from build123d import *

# Parameters (mm, degrees)
SKETCH_1_W          = 290
SKETCH_1_H          = 150
EXTRUDE_1_DEPTH     = 5
CUT_EXTRUDE_2_REACH = 165.325
SKETCH_5_R          = 27.5
SKETCH_5_R_2        = 2.6
FILLET_1_R          = 10
SKETCH_6_R          = 2.75
CUT_EXTRUDE_3_DEPTH = 10
SKETCH_7_R          = 1.6
CUT_EXTRUDE_4_DEPTH = 10


with BuildPart() as part:
    # 草图1 → 凸台-拉伸1 (new body)
    with BuildSketch(Plane.XY):
        Rectangle(SKETCH_1_W, SKETCH_1_H)
    extrude(amount=EXTRUDE_1_DEPTH)

    # 草图5 → 切除-拉伸2 (cut, up to next)
    with BuildSketch(Plane(origin=(0, 0, 0), x_dir=(-1, 0, 0), z_dir=(0, 0, -1)), mode=Mode.PRIVATE) as cut_extrude_2_sk1:
        Circle(SKETCH_5_R)
    cut_extrude_2_tool1 = extrude(cut_extrude_2_sk1.sketch, amount=-CUT_EXTRUDE_2_REACH, mode=Mode.PRIVATE) & part.part
    # 草图5 → 切除-拉伸2 (cut, up to next)
    with BuildSketch(Plane(origin=(0, 0, 0), x_dir=(-1, 0, 0), z_dir=(0, 0, -1)), mode=Mode.PRIVATE) as cut_extrude_2_sk2:
        with Locations((23.864853865, 23.864853865)):
            Circle(SKETCH_5_R_2)
    cut_extrude_2_tool2 = extrude(cut_extrude_2_sk2.sketch, amount=-CUT_EXTRUDE_2_REACH, mode=Mode.PRIVATE) & part.part
    # 草图5 → 切除-拉伸2 (cut, up to next)
    with BuildSketch(Plane(origin=(0, 0, 0), x_dir=(-1, 0, 0), z_dir=(0, 0, -1)), mode=Mode.PRIVATE) as cut_extrude_2_sk3:
        with Locations((0, 33.75)):
            Circle(SKETCH_5_R_2)
    cut_extrude_2_tool3 = extrude(cut_extrude_2_sk3.sketch, amount=-CUT_EXTRUDE_2_REACH, mode=Mode.PRIVATE) & part.part
    # 草图5 → 切除-拉伸2 (cut, up to next)
    with BuildSketch(Plane(origin=(0, 0, 0), x_dir=(-1, 0, 0), z_dir=(0, 0, -1)), mode=Mode.PRIVATE) as cut_extrude_2_sk4:
        with Locations((-23.864853865, 23.864853865)):
            Circle(SKETCH_5_R_2)
    cut_extrude_2_tool4 = extrude(cut_extrude_2_sk4.sketch, amount=-CUT_EXTRUDE_2_REACH, mode=Mode.PRIVATE) & part.part
    # 草图5 → 切除-拉伸2 (cut, up to next)
    with BuildSketch(Plane(origin=(0, 0, 0), x_dir=(-1, 0, 0), z_dir=(0, 0, -1)), mode=Mode.PRIVATE) as cut_extrude_2_sk5:
        with Locations((-33.75, 0)):
            Circle(SKETCH_5_R_2)
    cut_extrude_2_tool5 = extrude(cut_extrude_2_sk5.sketch, amount=-CUT_EXTRUDE_2_REACH, mode=Mode.PRIVATE) & part.part
    # 草图5 → 切除-拉伸2 (cut, up to next)
    with BuildSketch(Plane(origin=(0, 0, 0), x_dir=(-1, 0, 0), z_dir=(0, 0, -1)), mode=Mode.PRIVATE) as cut_extrude_2_sk6:
        with Locations((-23.864853865, -23.864853865)):
            Circle(SKETCH_5_R_2)
    cut_extrude_2_tool6 = extrude(cut_extrude_2_sk6.sketch, amount=-CUT_EXTRUDE_2_REACH, mode=Mode.PRIVATE) & part.part
    # 草图5 → 切除-拉伸2 (cut, up to next)
    with BuildSketch(Plane(origin=(0, 0, 0), x_dir=(-1, 0, 0), z_dir=(0, 0, -1)), mode=Mode.PRIVATE) as cut_extrude_2_sk7:
        with Locations((0, -33.75)):
            Circle(SKETCH_5_R_2)
    cut_extrude_2_tool7 = extrude(cut_extrude_2_sk7.sketch, amount=-CUT_EXTRUDE_2_REACH, mode=Mode.PRIVATE) & part.part
    # 草图5 → 切除-拉伸2 (cut, up to next)
    with BuildSketch(Plane(origin=(0, 0, 0), x_dir=(-1, 0, 0), z_dir=(0, 0, -1)), mode=Mode.PRIVATE) as cut_extrude_2_sk8:
        with Locations((23.864853865, -23.864853865)):
            Circle(SKETCH_5_R_2)
    cut_extrude_2_tool8 = extrude(cut_extrude_2_sk8.sketch, amount=-CUT_EXTRUDE_2_REACH, mode=Mode.PRIVATE) & part.part
    # 草图5 → 切除-拉伸2 (cut, up to next)
    with BuildSketch(Plane(origin=(0, 0, 0), x_dir=(-1, 0, 0), z_dir=(0, 0, -1)), mode=Mode.PRIVATE) as cut_extrude_2_sk9:
        with Locations((33.75, 0)):
            Circle(SKETCH_5_R_2)
    cut_extrude_2_tool9 = extrude(cut_extrude_2_sk9.sketch, amount=-CUT_EXTRUDE_2_REACH, mode=Mode.PRIVATE) & part.part
    add(cut_extrude_2_tool1.solids().sort_by_distance((0, 0, 0))[0], mode=Mode.SUBTRACT)
    add(cut_extrude_2_tool2.solids().sort_by_distance((-23.864854, 23.864854, 0))[0], mode=Mode.SUBTRACT)
    add(cut_extrude_2_tool3.solids().sort_by_distance((0, 33.75, 0))[0], mode=Mode.SUBTRACT)
    add(cut_extrude_2_tool4.solids().sort_by_distance((23.864854, 23.864854, 0))[0], mode=Mode.SUBTRACT)
    add(cut_extrude_2_tool5.solids().sort_by_distance((33.75, 0, 0))[0], mode=Mode.SUBTRACT)
    add(cut_extrude_2_tool6.solids().sort_by_distance((23.864854, -23.864854, 0))[0], mode=Mode.SUBTRACT)
    add(cut_extrude_2_tool7.solids().sort_by_distance((0, -33.75, 0))[0], mode=Mode.SUBTRACT)
    add(cut_extrude_2_tool8.solids().sort_by_distance((-23.864854, -23.864854, 0))[0], mode=Mode.SUBTRACT)
    add(cut_extrude_2_tool9.solids().sort_by_distance((-33.75, 0, 0))[0], mode=Mode.SUBTRACT)

    # 圆角1
    fillet_1_edges = [part.edges().sort_by_distance(p)[0] for p in [
        (145, -75, 2.5),
        (-145, -75, 2.5),
        (-145, 75, 2.5),
        (145, 75, 2.5),
    ]]
    fillet(fillet_1_edges, radius=FILLET_1_R)

    # 草图6 → 切除-拉伸3 (cut)
    with BuildSketch(Plane(origin=(0, 0, 0), x_dir=(-1, 0, 0), z_dir=(0, 0, -1))):
        with Locations((110, -16)):
            Circle(SKETCH_6_R)
        with Locations((-110, -16)):
            Circle(SKETCH_6_R)
        with Locations((-110, 16)):
            Circle(SKETCH_6_R)
        with Locations((110, 16)):
            Circle(SKETCH_6_R)
    extrude(amount=-CUT_EXTRUDE_3_DEPTH, mode=Mode.SUBTRACT)

    # 草图7 → 切除-拉伸4 (cut)
    with BuildSketch(Plane(origin=(0, 0, 0), x_dir=(-1, 0, 0), z_dir=(0, 0, -1))):
        with Locations((-135, 65)):
            Circle(SKETCH_7_R)
        with Locations((-115, 65)):
            Circle(SKETCH_7_R)
        with Locations((105, 65)):
            Circle(SKETCH_7_R)
        with Locations((125, 65)):
            Circle(SKETCH_7_R)
        with Locations((105, -65)):
            Circle(SKETCH_7_R)
        with Locations((125, -65)):
            Circle(SKETCH_7_R)
        with Locations((-135, -65)):
            Circle(SKETCH_7_R)
        with Locations((-115, -65)):
            Circle(SKETCH_7_R)
    extrude(amount=-CUT_EXTRUDE_4_DEPTH, mode=Mode.SUBTRACT)


solid = part.part
Read the model definition and answer for the solid it produces. Units are mm, in the model's axes. Round coordinates to 2 decimals unless told otherwise and drop trailing zeros. Write each loop counter-clockwise with the first axis right and the second up, starting at its lowest first coordinate (ties: lowest second). Pieces come first, ordered by that corner, then holes. Notation, with made-up numbers: M 53.25,18 L 96.25,18 A9 cw 96.25,30 Z; hole C 64,0.25 d11. An arc over 180 degrees is marked long. Use a Markdown table: item, result.
1) Straight lines are drawn through the part: line 1 along Y through (x, z) = (-105, 1.2); line 2 along Y through (x, z) = (110, 1.55); line 3 along X through (y, z) = (65, 2.55). For each, find the intervals that lie inside material, in ascending order. Write a range as [from, to].
Answers follow:
| item | result |
|---|---|
| line 1 | y = [-75, -66.6], [-63.4, 63.4], [66.6, 75] |
| line 2 | y = [-75, -18.75], [-13.25, 13.25], [18.75, 75] |
| line 3 | x = [-145, -126.6], [-123.4, -106.6], [-103.4, 113.4], [116.6, 133.4], [136.6, 145] |
2) The part is cut by section A-A (x = 16). Write down the section's boundary in (y, z).
Answers follow:
| item | result |
|---|---|
| outline | M -75,0 L -22.37,0 L -22.37,5 L -75,5 Z; M 22.37,0 L 75,0 L 75,5 L 22.37,5 Z |
3) The part is cut by section B-B (z = 2.7). Give the number of separate pieces and of enclosed holes in the cut face, plus the area to 3 significant figures.
Answers follow:
| item | result |
|---|---|
| separate pieces | 1 |
| enclosed holes | 21 |
| area | 40,700 mm2 |
4) For a pull along X with two mould halves and no side action, classify faces 1 (the flat face through (145, -1, 2)), 2 (the cylindrical face through (5.961, -26.846, 2.465)), 3 (the flat face through (30, 1, 5)) as pulls with the +X half, pulls with the -X half, needs draft (parallel to the pull), parting line crosses it, or undercut.
Answers follow:
| item | result |
|---|---|
| face 1 | pulls with the +X half |
| face 2 | undercut |
| face 3 | needs draft |
